Work out the finished part from the listing and answer in its coordinate system (mm). A direction names the side the tool comes from. Give positions to 0.01 mm unless a question says otherwise; leave off trailing zeros. Write each loop counter-clockwise with the first axis right and the second up, starting at its lowest first coordinate (ties: lowest second). Pieces come first, ordered by that corner, then holes.
1) Find section A-A (x = 0). Determine the outline of the cut face in (y, z).
2) Find section C-C (z = 61). Determine the outline of the cut face in (x, y), plus the area to 3 significant figures.
3) Straight lines are drawn through the part: probe 1 along Y at (x, z) = (0, 67.75); probe 2 along Y at (x, z) = (-0.25, 17); probe 3 along X at (y, z) = (-0.75, 64.5). For each, find the intervals that lie inside material, in ascending order.
4) Determine the mould class of faces 4 (the face through (2, 0, 70)), 5 (the face through (-0.867, -3.905, 34.51)), 6 (the face through (-0.29, -1.32, 65.07)) for opening direction X: pulls with the +X half, pulls with the -X half, needs draft (parallel to the pull), parting line crosses it, or undercut.
5) A tool of negligible diameter and unlimited length cuts with its end or side. For faces 1 (the face through (-0.29, 1.32, 4.93)), 2 (the face through (2, 0, 0)), 3 (the face through (0, 0, 60)), from which of +Z, -Z, +X, -X, +Y, -Y can it reach the whole face along a straight path? Write none if from no direction.
6) Given pin 1 Ø1.5 at (x, z) = (2.5, 58) entering from +Y; pin 2 Ø0.8 at (x, y) = (0, 0.5) entering from +Z; pin 3 Ø2 at (y, z) = (-1, 32) entering from -X; pin 4 Ø2 at (y, z) = (-2.5, 45) entering from -X, each flat-ended and moving along its own axis, determine where each tip first touches the part or whether it passes through.
7) Find section D-D (z = 51). Determine the outline of the cut face in (x, y).
```python
from build123d import *

# Parameters (mm, degrees)
SKETCH_R        = 4
PAD_DEPTH       = 70
SKETCH001_R     = 1.35
POCKET_DEPTH    = 10
SKETCH002_R     = 1.35
POCKET001_DEPTH = 10


with BuildPart() as part:
    # Sketch → Pad (new body)
    with BuildSketch(Plane.XY):
        Circle(SKETCH_R)
    extrude(amount=PAD_DEPTH)

    # Sketch001 → Pocket (cut)
    with BuildSketch(Plane.XY.offset(70)):
        Circle(SKETCH001_R)
    extrude(amount=-POCKET_DEPTH, mode=Mode.SUBTRACT)

    # Sketch002 → Pocket001 (cut)
    with BuildSketch(Plane(origin=(0, 0, 0), x_dir=(1, 0, 0), z_dir=(0, 0, -1))):
        Circle(SKETCH002_R)
    extrude(amount=-POCKET001_DEPTH, mode=Mode.SUBTRACT)


solid = part.part
```
Results:
1. outline: (-4, 0) - (-1.35, 0) - (-1.35, 10) - (1.35, 10) - (1.35, 0) - (4, 0) - (4, 70) - (1.35, 70) - (1.35, 60) - (-1.35, 60) - (-1.35, 70) - (-4, 70) - close
2. outline: circle Ø8 at (0, 0); hole circle Ø2.7 at (0, 0)
2. area: 44.5 mm2
3. probe 1: y = -4 to -1.35, 1.35 to 4
3. probe 2: y = -3.99 to 3.99
3. probe 3: x = -3.93 to -1.12, 1.12 to 3.93
4. face 4: needs draft
4. face 5: parting line crosses it
4. face 6: undercut
5. face 1: -Z
5. face 2: -Z, +X, -X, +Y, -Y
5. face 3: +Z
6. pin 1: stops at y = 3.6
6. pin 2: stops at z = 60
6. pin 3: stops at x = -4
6. pin 4: stops at x = -3.71
7. outline: circle Ø8 at (0, 0)
